Verification items for the finished model (mm, model axes). Give positions to 0.01 mm unless a question says otherwise; leave off trailing zeros. Loops run counter-clockwise (first coordinate to the right, second up) from the corner with the lowest first, then second, coordinate; pieces in that order, holes last. Notation, with made-up numbers: (-39, 45.25) - (-27, 45.25) arc R20 ccw to (-27, 82.25) - close; hole circle Ø3 at (2, -32). An arc over 180 degrees is marked (long way). Use one line per item in the form item = value.
```python
from build123d import *

# Parameters (mm, degrees)
SKETCH_529_W           = 518
SKETCH_529_H           = 297
EXTRUDE_601_DEPTH      = 51
SKETCH_5_3_R           = 30
CUT_EXTRUDE_11_DEPTH   = 10
SKETCH_5_3_2_R         = 22.5
CUT_EXTRUDE_11_2_DEPTH = 25


with BuildPart() as part:
    # Sketch 529 → Extrude 601 (new body)
    with BuildSketch(Plane(origin=(0, 0, 0), x_dir=(1, 0, 0), z_dir=(0, 1, 0))):
        with Locations((184, -92)):
            Rectangle(SKETCH_529_W, SKETCH_529_H)
    extrude(amount=EXTRUDE_601_DEPTH)

    # Sketch 5_3 → Ложемент для КМЕ-11 (cut)
    with BuildSketch(Plane(origin=(0, 0, 0), x_dir=(1, 0, 0), z_dir=(0, 1, 0))):
        with Locations(Location((0, 0, 0), (0, 0, 270))):
            Circle(SKETCH_5_3_R)
        with Locations(Location((92, 0, 0), (0, 0, 270))):
            Circle(SKETCH_5_3_R)
        with Locations(Location((184, 0, 0), (0, 0, 270))):
            Circle(SKETCH_5_3_R)
        with Locations(Location((276, 0, 0), (0, 0, 270))):
            Circle(SKETCH_5_3_R)
        with Locations(Location((368, 0, 0), (0, 0, 270))):
            Circle(SKETCH_5_3_R)
        with Locations(Location((0, -92, 0), (0, 0, 270))):
            Circle(SKETCH_5_3_R)
        with Locations(Location((92, -92, 0), (0, 0, 270))):
            Circle(SKETCH_5_3_R)
        with Locations(Location((184, -92, 0), (0, 0, 270))):
            Circle(SKETCH_5_3_R)
        with Locations(Location((276, -92, 0), (0, 0, 270))):
            Circle(SKETCH_5_3_R)
        with Locations(Location((368, -92, 0), (0, 0, 270))):
            Circle(SKETCH_5_3_R)
        with Locations(Location((0, -184, 0), (0, 0, 270))):
            Circle(SKETCH_5_3_R)
        with Locations(Location((92, -184, 0), (0, 0, 270))):
            Circle(SKETCH_5_3_R)
        with Locations(Location((184, -184, 0), (0, 0, 270))):
            Circle(SKETCH_5_3_R)
        with Locations(Location((276, -184, 0), (0, 0, 270))):
            Circle(SKETCH_5_3_R)
        with Locations(Location((368, -184, 0), (0, 0, 270))):
            Circle(SKETCH_5_3_R)
    extrude(amount=CUT_EXTRUDE_11_DEPTH, mode=Mode.SUBTRACT)

    # Sketch 5_3 2 → Ложемент для КМЕ-11 (2) (cut)
    with BuildSketch(Plane.XZ):
        with Locations(Location((0, 0, 0), (0, 0, 270))):
            Circle(SKETCH_5_3_2_R)
        with Locations(Location((92, 0, 0), (0, 0, 270))):
            Circle(SKETCH_5_3_2_R)
        with Locations(Location((184, 0, 0), (0, 0, 270))):
            Circle(SKETCH_5_3_2_R)
        with Locations(Location((276, 0, 0), (0, 0, 270))):
            Circle(SKETCH_5_3_2_R)
        with Locations(Location((368, 0, 0), (0, 0, 270))):
            Circle(SKETCH_5_3_2_R)
        with Locations(Location((92, 92, 0), (0, 0, 270))):
            Circle(SKETCH_5_3_2_R)
        with Locations(Location((184, 92, 0), (0, 0, 270))):
            Circle(SKETCH_5_3_2_R)
        with Locations(Location((276, 92, 0), (0, 0, 270))):
            Circle(SKETCH_5_3_2_R)
        with Locations(Location((368, 92, 0), (0, 0, 270))):
            Circle(SKETCH_5_3_2_R)
        with Locations(Location((92, 184, 0), (0, 0, 270))):
            Circle(SKETCH_5_3_2_R)
        with Locations(Location((184, 184, 0), (0, 0, 270))):
            Circle(SKETCH_5_3_2_R)
        with Locations(Location((276, 184, 0), (0, 0, 270))):
            Circle(SKETCH_5_3_2_R)
        with Locations(Location((368, 184, 0), (0, 0, 270))):
            Circle(SKETCH_5_3_2_R)
        with Locations(Location((0, 92, 0), (0, 0, 270))):
            Circle(SKETCH_5_3_2_R)
        with Locations(Location((0, 184, 0), (0, 0, 270))):
            Circle(SKETCH_5_3_2_R)
    extrude(amount=-CUT_EXTRUDE_11_2_DEPTH, mode=Mode.SUBTRACT)


solid = part.part
```
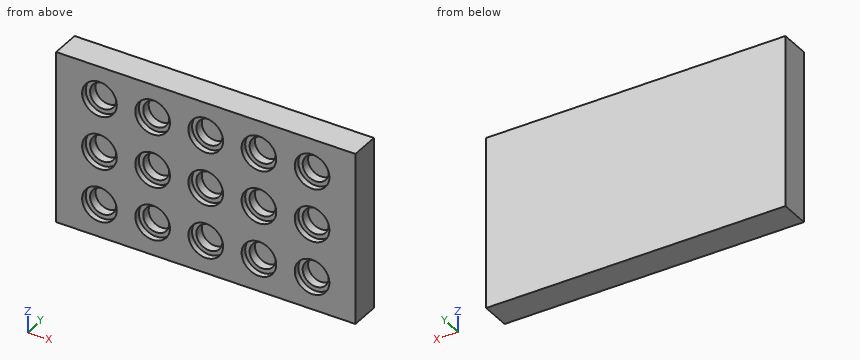
1. Section check B-B, the plane x = 169.5. Record the cut outline in (y, z), then the cut area to 3 significant figures.
Result set:
outline = (0, -56.5) - (51, -56.5) - (51, 240.5) - (0, 240.5) - (0, 210.26) - (10, 210.26) - (10, 201.2) - (25, 201.2) - (25, 166.8) - (10, 166.8) - (10, 157.74) - (0, 157.74) - (0, 118.26) - (10, 118.26) - (10, 109.2) - (25, 109.2) - (25, 74.8) - (10, 74.8) - (10, 65.74) - (0, 65.74) - (0, 26.26) - (10, 26.26) - (10, 17.2) - (25, 17.2) - (25, -17.2) - (10, -17.2) - (10, -26.26) - (0, -26.26) - close
area = 12,000 mm²
2. Scan lines: probe 1 along X at (y, z) = (3, 0); probe 2 along X at (y, z) = (17, 0); probe 3 along Z at (x, y) = (296, 4.5). Record each from-to range of solid material in increasing order.
Result set:
probe_1 = -75 to -30, 30 to 62, 122 to 154, 214 to 246, 306 to 338, 398 to 443
probe_2 = -75 to -22.5, 22.5 to 69.5, 114.5 to 161.5, 206.5 to 253.5, 298.5 to 345.5, 390.5 to 443
probe_3 = -56.5 to -22.36, 22.36 to 69.64, 114.36 to 161.64, 206.36 to 240.5
3. Section check A-A, the plane x = 92. Record the cut outline in (y, z), then the cut area to 3 significant figures.
Result set:
outline = (0, -56.5) - (51, -56.5) - (51, 240.5) - (0, 240.5) - (0, 214) - (10, 214) - (10, 206.5) - (25, 206.5) - (25, 161.5) - (10, 161.5) - (10, 154) - (0, 154) - (0, 122) - (10, 122) - (10, 114.5) - (25, 114.5) - (25, 69.5) - (10, 69.5) - (10, 62) - (0, 62) - (0, 30) - (10, 30) - (10, 22.5) - (25, 22.5) - (25, -22.5) - (10, -22.5) - (10, -30) - (0, -30) - close
area = 11,300 mm²
4. Depth check by flat-ended pin: pin 1 Ø13.5 at (x, z) = (365.5, 180) entering from -Y; pin 2 Ø1 at (x, z) = (195, 25.5) entering from -Y. Enter the tip coordinate at first touch or a pass-through.
Result set:
pin_1 = 25
pin_2 = 10
